Can you work these out from the model? Positions are in its coordinate system, mm. A direction names the side the tool comes from. Round coordinates to 2 decimals unless told otherwise and drop trailing zeros. Loops run counter-clockwise (first coordinate to the right, second up) from the corner with the lowest first, then second, coordinate; pieces in that order, holes last. Notation, with made-up numbers: M -4.5,21.5 L 48.5,21.5 A21 ccw 48.5,31.5 Z; hole C 34.25,-15 d10. An arc over 180 degrees is marked long. Return JSON: item names as keys, results as strings.
```python
from build123d import *

# Parameters (mm, degrees)
SKETCH1_W                   = 25.4
SKETCH1_H                   = 25.4
SKETCH1_W_2                 = 19.05
SKETCH1_H_2                 = 19.05
BASE_TUBE_DEPTH             = 38.1
INITIAL_10_HOLE_D           = 4.9149
F_10_HOLE_PATTERN_COUNT     = 4
F_10_HOLE_PATTERN_PITCH     = 12.7
F_10_HOLE_PATTERN_COL_COUNT = 4
F_10_HOLE_PATTERN_COL_PITCH = 12.7
CUT_EXTRUDE1_REACH          = 49.519
SKETCH8_R                   = 3.175


with BuildPart() as part:
    # Sketch1 → Base Tube (new, symmetric)
    with BuildSketch(Plane(origin=(0, 0, 0), x_dir=(0, 0, -1), z_dir=(1, 0, 0))):
        Rectangle(SKETCH1_W, SKETCH1_H)
        Rectangle(SKETCH1_W_2, SKETCH1_H_2, mode=Mode.SUBTRACT)
    extrude(amount=BASE_TUBE_DEPTH, both=True)

    # Initial #10 Hole (through all)
    with Locations(Plane(origin=(0, 12.7, 0), x_dir=(1, 0, 0), z_dir=(0, 1, 0))):
        with Locations((0, 0)):
            initial_10_hole = Hole(INITIAL_10_HOLE_D / 2)

    # #10 Hole Pattern: Initial #10 Hole ×4
    with Locations(*[(i * F_10_HOLE_PATTERN_PITCH, 0, 0) for i in range(1, F_10_HOLE_PATTERN_COUNT)]):
        add(initial_10_hole, mode=Mode.SUBTRACT)

    # #10 Hole Pattern col: Initial #10 Hole ×4
    with Locations(*[(-i * F_10_HOLE_PATTERN_COL_PITCH, 0, 0) for i in range(1, F_10_HOLE_PATTERN_COL_COUNT)]):
        add(initial_10_hole, mode=Mode.SUBTRACT)

    # Sketch8 → Cut-Extrude1 (cut, up to next)
    with BuildSketch(Plane.XY.offset(12.7), mode=Mode.PRIVATE) as cut_extrude1_sk1:
        with Locations((-0.402530278, -1.19507)):
            Circle(SKETCH8_R)
    cut_extrude1_tool1 = extrude(cut_extrude1_sk1.sketch, amount=-CUT_EXTRUDE1_REACH, mode=Mode.PRIVATE) & part.part
    add(cut_extrude1_tool1.solids().sort_by_distance((-0.40253, -1.19507, 12.7))[0], mode=Mode.SUBTRACT)


solid = part.part
```
Q1. Thinking about a two-plate mould opening in Y: for faces 4 (the cylindrical face through (35.643, 11.09, 0.054)), 5 (the flat face through (1, 12.7, -3)), 6 (the flat face through (1, 9.525, -4)), which applies, pulls with the +Y half, pulls with the -Y half, needs draft (parallel to the pull), parting line crosses it, or undercut?
Results:
{"face 4": "needs draft", "face 5": "pulls with the +Y half", "face 6": "undercut"}
Q2. Suppose I cut it at C-C, the plane x = 25.4. Please give me the cut outline in (y, z) (3 decimals), plus the area to 3 significant figures.
Results:
{"outline": "M -12.7,-12.7 L 12.7,-12.7 L 12.7,-2.457 L 9.525,-2.457 L 9.525,-9.525 L -9.525,-9.525 L -9.525,-2.457 L -12.7,-2.457 Z; M -12.7,2.457 L -9.525,2.457 L -9.525,9.525 L 9.525,9.525 L 9.525,2.457 L 12.7,2.457 L 12.7,12.7 L -12.7,12.7 Z", "area": "251 mm2"}
Q3. I'm going to push flat-ended pins straight in: pin 1 Ø3 at (x, z) = (15, 0.5) entering from +Y; pin 2 Ø4 at (x, z) = (-25.4, 0) entering from -Y. Where does each tip first touch, or does it pass through?
Results:
{"pin 1": "stops at y = 12.7", "pin 2": "passes through"}
Q4. On a 3-axis mill with a long thin cutter (end or side, diameter ignored), from which of +Z, -Z, +X, -X, +Y, -Y can I reach the whole of each face in a straight line? I mean faces 1 (the cylindrical face through (-35.643, 11.09, -0.054)), 2 (the cylindrical face through (2.626, -0.241, 11.135)), 3 (the flat face through (1, 2, 9.525)). Say none if no direction works.
Results:
{"face 1": "-X, +Y, -Y", "face 2": "+Z", "face 3": "+X, -X"}
Q5. Suppose I cut it at B-B, the plane y = 10.5. Please give me the cut outline in (x, z), plus the area to 3 significant figures.
Results:
{"outline": "M -38.1,-12.7 L 38.1,-12.7 L 38.1,-2.46 A2.46 cw 38.1,2.46 L 38.1,12.7 L -38.1,12.7 L -38.1,2.46 A2.46 cw -38.1,-2.46 Z; hole C -25.4,0 d4.91; hole C -12.7,0 d4.91; hole C 0,0 d4.91; hole C 12.7,0 d4.91; hole C 25.4,0 d4.91", "area": "1,820 mm2"}
Q6. If I drill on line 1 along Z through (x, y) = (18, 6.75) (3 decimals); line 2 along Z through (x, y) = (-25.4, 11.9), over which ranges is the centre line in solid material (lowest first)?
Results:
{"line 1": "z = -12.7 to -9.525, 9.525 to 12.7", "line 2": "z = -12.7 to -2.46, 2.46 to 12.7"}
Q7. Suppose I cut it at A-A, the plane x = 8.5. Please give me the cut outline in (y, z) (3 decimals), plus the area to 3 significant figures.
Results:
{"outline": "M -12.7,-12.7 L 12.7,-12.7 L 12.7,12.7 L -12.7,12.7 Z; hole M -9.525,-9.525 L 9.525,-9.525 L 9.525,9.525 L -9.525,9.525 Z", "area": "282 mm2"}
Q8. Suppose I cut it at D-D, the plane z = -7.25. Please give me the cut outline in (x, y) (3 decimals), plus the area to 3 significant figures.
Results:
{"outline": "M -38.1,-12.7 L 38.1,-12.7 L 38.1,-9.525 L -38.1,-9.525 Z; M -38.1,9.525 L 38.1,9.525 L 38.1,12.7 L -38.1,12.7 Z", "area": "484 mm2"}
